Check sheet for the modelled part. Datum: model origin and axes. Units: mm. A direction names the side the tool comes from. Round coordinates to 2 decimals unless told otherwise and drop trailing zeros. Order: outer loops, then holes, each group sorted by start corner. A loop starts at its lowest first (then second) coordinate and runs counter-clockwise, first axis right, second up. Notation, with made-up numbers: M 14,51.25 L 58,51.25 A25 ccw 58,70.25 Z; hole C -9,-2 d1. An arc over 180 degrees is marked long. One line per item, written item: value. Start each with the question number.
(1) Release check for a two-part mould opening along X. For faces 4 (the face through (0, 0, 55)), 5 (the face through (-140, 0, 65)), 6 (the face through (-2, 0, 100)), 7 (the face through (140, 0, 65)) record: released by +X, released by -X, zero draft, split by the parting line, or undercut.
(2) Thickness scan on L1, parallel to X at y = 2, z = 65; L2, parallel to Z at x = 0, y = -2; L3, parallel to Z at x = 54.5, y = 22. Record the ranges inside material, lowest first.
(3) Cross-section at D-D, the plane z = 9. Enter the section's corners in (x, y).
(4) Depth check by flat-ended pin: pin 1 Ø12 at (x, z) = (0, 65) entering from -Y; pin 2 Ø15.5 at (x, y) = (-46, 6.5) entering from -Z; pin 3 Ø5 at (y, z) = (-18, -5.5) entering from -X; pin 4 Ø15.5 at (y, z) = (-12, -50.5) entering from +X. Enter the tip coordinate at first touch or a pass-through.
(5) Cross-section at B-B, the plane x = 0. Enter the section's corners in (y, z), and give its area (3 significant figures).
(6) Cross-section at A-A, the plane y = -7.5. Enter the section's corners in (x, z).
(7) Access from +Z, -Z, +X, -X, +Y, -Y to the whole of each face (thin tool, end or side, straight path). Record for faces 1 (the face through (-10, 0, -36)), 2 (the face through (-2, -25.5, 43)), 3 (the face through (10, 0, -34)).
(8) Cross-section at C-C, the plane z = 59. Enter the section's corners in (x, y).
from build123d import *

# Parameters (mm, degrees)
EXTRUDE_1_DEPTH          = 25.5
CUT_EXTRUDE_1_DEPTH      = 174.925990007
CUT_EXTRUDE_1_DEPTH_BACK = 174.925990007
SKETCH_2_R               = 10


with BuildPart() as part:
    # Эскиз1 → Бобышка-Вытянуть1 (new, symmetric)
    with BuildSketch(Plane(origin=(0, 0, 0), x_dir=(1, 0, 0), z_dir=(0, 1, 0))):
        Polygon((10, 100), (-10, 100), (-10, -30), (-140, -30), (-140, -100), (140, -100), (140, -30), (10, -30), align=None)
    extrude(amount=EXTRUDE_1_DEPTH, both=True)

    # Эскиз2 → Вырез-Вытянуть1 (cut, two sides: drawn at the far end of the back side and taken through both)
    with BuildSketch(Plane(origin=(0, 0, 0), x_dir=(1, 0, 0), z_dir=(0, 1, 0)).offset(-CUT_EXTRUDE_1_DEPTH_BACK)):
        with Locations(Location((0, -65, 0), (0, 0, 270))):
            Circle(SKETCH_2_R)
    extrude(amount=CUT_EXTRUDE_1_DEPTH + CUT_EXTRUDE_1_DEPTH_BACK, mode=Mode.SUBTRACT)


solid = part.part
Values found:
1. face 4: undercut
1. face 5: released by -X
1. face 6: zero draft
1. face 7: released by +X
2. L1: -140 to -10, 10 to 140
2. L2: -100 to 55, 75 to 100
2. L3: 30 to 100
3. outline: M -10,-25.5 L 10,-25.5 L 10,25.5 L -10,25.5 Z
4. pin 1: through
4. pin 2: z = 30
4. pin 3: x = -10
4. pin 4: x = 10
5. outline: M -25.5,-100 L 25.5,-100 L 25.5,55 L -25.5,55 Z; M -25.5,75 L 25.5,75 L 25.5,100 L -25.5,100 Z
5. area: 9,180 mm^2
6. outline: M -140,30 L -10,30 L -10,-100 L 10,-100 L 10,30 L 140,30 L 140,100 L -140,100 Z; hole C 0,65 d20
7. face 1: -Z, -X, +Y, -Y
7. face 2: +Z, -Z, +X, -X, -Y
7. face 3: -Z, +X, +Y, -Y
8. outline: M -140,-25.5 L -8,-25.5 L -8,25.5 L -140,25.5 Z; M 8,-25.5 L 140,-25.5 L 140,25.5 L 8,25.5 Z
